from build123d import *

# Parameters (mm, degrees)
F0_R     = 69.542462
F1_DEPTH = 101.6
F2_W     = 50.384016
F2_H     = 45.657624
F3_DEPTH = 50.8
F5_D     = 25.4
F7_D     = 25.4


with BuildPart() as f1:
    # F0 (on Top) → F1 (new body)
    with BuildSketch(Plane.XY):
        Circle(F0_R)
    extrude(amount=F1_DEPTH)

    # F2 (on face) → F3 (join)
    with BuildSketch(Plane.XY.offset(101.6)):
        with Locations((-2.197395, -3.927665)):
            Rectangle(F2_W, F2_H)
    extrude(amount=F3_DEPTH)

    # F5 (through all)
    with Locations(Plane(origin=(0, 18.901147, 0), x_dir=(-1, 0, 0), z_dir=(0, 1, 0))):
        with Locations((0, 133.62363)):
            Hole(F5_D / 2)

    # F7 (through all)
    with Locations(Plane.XY.offset(101.6)):
        with Locations((41.455068, 7.525192)):
            Hole(F7_D / 2)


solid = f1.part
For this review, take the finished solid that the model builds, in its own axes (mm). A direction names the side the tool comes from. Coordinates: 2 decimals unless noted, no trailing zeros. Order: outer loops, then holes, each group sorted by start corner. A loop starts at its lowest first (then second) coordinate and runs counter-clockwise, first axis right, second up. Notation, with made-up numbers: (14, 6) -> (38, 6) arc R15 ccw to (38, 32) -> close; hole circle Ø5 at (-30, -19). An arc over 180 degrees is marked (long way). Return JSON: item names as keys, results as strings.
1. For line 1 (Z direction, x = 0, y = -2); line 2 (Z direction, x = 39, y = 52.5); line 3 (Y direction, x = 36, z = 93.5), list the stretches that pass through material, from the lowest coordinate up. Write a range as from..to.
Answer block:
{"line 1": "0..120.92, 146.32..152.4", "line 2": "0..101.6", "line 3": "-59.5..-3.94, 18.99..59.5"}
2. We need section A-A on y = 0. Write out the cut boundary in (x, z), and give its area (3 significant figures).
Answer block:
{"outline": "(-69.54, 0) -> (31.22, 0) -> (31.22, 101.6) -> (22.99, 101.6) -> (22.99, 152.4) -> (-27.39, 152.4) -> (-27.39, 101.6) -> (-69.54, 101.6) -> close; (51.69, 0) -> (69.54, 0) -> (69.54, 101.6) -> (51.69, 101.6) -> close; hole circle Ø25.4 at (0, 133.62)", "area": "14,100 mm²"}
3. Machinability: for faces 4 (the flat face through (-3, -26.756, 121)), 5 (the flat face through (-3, 18.901, 121)), 6 (the flat face through (22.995, -4, 127)), 7 (the flat face through (-1, 1, 0)), 8 (the cylindrical face through (29.34, 11.34, 50.09)), which of the approach directions +Z, -Z, +X, -X, +Y, -Y give a long, thin tool a straight path to every point of the face, cutting with its end or side? Answer none if there is none.
Answer block:
{"face 4": "+Z, +X, -X, -Y", "face 5": "+Z, +X, -X, +Y", "face 6": "+Z, +X, +Y, -Y", "face 7": "-Z, +X, -X, +Y, -Y", "face 8": "+Z, -Z"}
4. For pin 1 Ø4 at (x, z) = (51.5, 26.5) entering from -Y; pin 2 Ø25 at (x, z) = (-4, 115) entering from -Y; pin 3 Ø10 at (y, z) = (44.5, 92) entering from -X; pin 4 Ø1 at (x, y) = (26, 52.5) entering from -Z, all flat-tipped, find the tip position at first contact; note any pin that passes through.
Answer block:
{"pin 1": "y = -48.85", "pin 2": "y = -26.76", "pin 3": "x = -57.24", "pin 4": "z = 0"}
5. We need section D-D on x = 31. Write out the cut boundary in (y, z).
Answer block:
{"outline": "(-62.25, 0) -> (0.32, 0) -> (0.32, 101.6) -> (-62.25, 101.6) -> close; (14.74, 0) -> (62.25, 0) -> (62.25, 101.6) -> (14.74, 101.6) -> close"}
6. We need section C-C on z = 125. Write out the cut boundary in (x, y), and give its area (3 significant figures).
Answer block:
{"outline": "(-27.39, -26.76) -> (-9.32, -26.76) -> (-9.32, 18.9) -> (-27.39, 18.9) -> close; (9.32, -26.76) -> (22.99, -26.76) -> (22.99, 18.9) -> (9.32, 18.9) -> close", "area": "1,450 mm²"}
7. We need section B-B on x = 0. Write out the cut boundary in (y, z), and give its area (3 significant figures).
Answer block:
{"outline": "(-69.54, 0) -> (69.54, 0) -> (69.54, 101.6) -> (18.9, 101.6) -> (18.9, 120.92) -> (-26.76, 120.92) -> (-26.76, 101.6) -> (-69.54, 101.6) -> close; (-26.76, 146.32) -> (18.9, 146.32) -> (18.9, 152.4) -> (-26.76, 152.4) -> close", "area": "15,300 mm²"}
8. The part is to be moulded in two halves that separate along X. For faces 1 (the cylindrical face through (-2.753, -4.247, 121.226)), 2 (the cylindrical face through (-15.075, -67.889, 50.089)), 3 (the flat face through (-27.389, -4, 127)), say which applies: +X half, -X half, draft (parallel to the pull), parting line (faces both ways), or undercut.
Answer block:
{"face 1": "undercut", "face 2": "parting line", "face 3": "-X half"}
